from build123d import *

# Parameters (mm, degrees)
SKETCH1_W           = 15.875
SKETCH1_H           = 34.925
BOSS_EXTRUDE1_DEPTH = 6.35
SKETCH3_W           = 15.875
SKETCH3_H           = 18.415
BOSS_EXTRUDE2_DEPTH = 7.9375
SKETCH4_R           = 26.9875
CUT_EXTRUDE2_DEPTH  = 3.2385
SKETCH5_W           = 15.875
SKETCH5_H           = 8.68045
BOSS_EXTRUDE3_DEPTH = 3.175
FILLET1_R           = 0.254
FILLET2_R           = 3.175
SKETCH6_W           = 15.875
SKETCH6_H           = 6.35
BOSS_EXTRUDE4_DEPTH = 4.7625
SKETCH7_W           = 15.875
SKETCH7_H           = 3.175
BOSS_EXTRUDE5_DEPTH = 6.604
CUT_EXTRUDE3_REACH  = 48.174
SKETCH8_R           = 1.651


with BuildPart() as part:
    # Sketch1 → Boss-Extrude1 (new body)
    with BuildSketch(Plane.XY):
        with Locations((7.9375, 17.4625)):
            Rectangle(SKETCH1_W, SKETCH1_H)
    extrude(amount=BOSS_EXTRUDE1_DEPTH)

    # Sketch3 → Boss-Extrude2 (add)
    with BuildSketch(Plane.XY.offset(6.35)):
        with Locations((7.9375, 25.7175)):
            Rectangle(SKETCH3_W, SKETCH3_H)
    extrude(amount=BOSS_EXTRUDE2_DEPTH)

    # Sketch4 → Cut-Extrude2 (cut, symmetric)
    with BuildSketch(Plane(origin=(0, 28.42895, 0), x_dir=(-1, 0, 0), z_dir=(0, -1, 0))):
        with Locations((-7.9375, -36.4998)):
            Circle(SKETCH4_R)
    extrude(amount=CUT_EXTRUDE2_DEPTH, both=True, mode=Mode.SUBTRACT)

    # Sketch5 → Boss-Extrude3 (add)
    with BuildSketch(Plane.XY.offset(14.2875)):
        with Locations((7.9375, 20.850225)):
            Rectangle(SKETCH5_W, SKETCH5_H)
    extrude(amount=BOSS_EXTRUDE3_DEPTH)

    # Fillet1
    fillet1_edges = [part.edges().sort_by_distance(p)[0] for p in [
        (0, 33.296225, 14.2875),
        (15.875, 33.296225, 14.2875),
        (7.9375, 31.66745, 14.2875),
        (15.875, 28.42895, 10.705978065),
        (0, 28.42895, 10.705978065),
        (0, 25.19045, 14.084239033),
        (15.875, 25.19045, 14.084239033),
        (0, 31.66745, 12.496739033),
        (15.875, 31.66745, 12.496739033),
        (7.9375, 25.19045, 17.4625),
    ]]
    fillet(fillet1_edges, radius=FILLET1_R)

    # Fillet2
    fillet2_edges = [part.edges().sort_by_distance(p)[0] for p in [
        (7.9375, 16.51, 6.35),
    ]]
    fillet(fillet2_edges, radius=FILLET2_R)

    # Sketch6 → Boss-Extrude4 (add)
    with BuildSketch(Plane.XZ):
        with Locations((7.9375, 3.175)):
            Rectangle(SKETCH6_W, SKETCH6_H)
    extrude(amount=BOSS_EXTRUDE4_DEPTH)

    # Sketch7 → Boss-Extrude5 (add)
    with BuildSketch(Plane.XY.offset(6.35)):
        with Locations((7.9375, -3.175)):
            Rectangle(SKETCH7_W, SKETCH7_H)
    extrude(amount=BOSS_EXTRUDE5_DEPTH)

    # Sketch8 → Cut-Extrude3 (cut, up to next)
    with BuildSketch(Plane.XZ.offset(4.7625), mode=Mode.PRIVATE) as cut_extrude3_sk1:
        with Locations(Location((7.9375, 9.8552, 0), (0, 0, 270))):
            Circle(SKETCH8_R)
    cut_extrude3_tool1 = extrude(cut_extrude3_sk1.sketch, amount=-CUT_EXTRUDE3_REACH, mode=Mode.PRIVATE) & part.part
    add(cut_extrude3_tool1.solids().sort_by_distance((7.9375, -4.7625, 9.8552))[0], mode=Mode.SUBTRACT)


solid = part.part
Can you work these out from the model? Positions are in its coordinate system, mm. A direction names the side the tool comes from. Round coordinates to 2 decimals unless told otherwise and drop trailing zeros. Loops run counter-clockwise (first coordinate to the right, second up) from the corner with the lowest first, then second, coordinate; pieces in that order, holes last. Notation, with made-up numbers: (70, -11.75) - (118, -11.75) arc R15 ccw to (118, 14.25) - close; hole circle Ø11 at (-5.75, 42). An arc over 180 degrees is marked (long way). Write item = value, one per line. Start each with the question number.
(1) If I drill on probe 1 along Y at (x, z) = (2.5, 10.25) (1 decimal); probe 2 along Y at (x, z) = (12.75, 14) (3 decimals); probe 3 along Y at (x, z) = (10.5, 15.5), over which ranges is the centre line in solid material (lowest first)? Write a range as [from, to].
(2) If we section it at A-A (z = 13.5): Please give me the cut outline in (x, y) (3 decimals), and give its area (3 significant figures).
(3) For P1, Ø3.5, axis at x = 9.5, y = 33, coming from the +Z side; P2, Ø1.6, axis at x = 6, y = -3.5, coming from the +Z side; P3, Ø10, axis at y = 2.5, z = 10, coming from the +X side (3 decimals); P4, Ø1, axis at x = 4, y = -0.5, coming from the +Z side, each with a flat end and sliding along its axis, tell me the tip position at first contact or that it passes through.
(4) If we section it at D-D (z = 16): Please give me the cut outline in (x, y) (3 decimals).
(5) For faces 1 (the face through (8, 6, 6.35)), 2 (the face through (8, 33, 14.288)), 3 (the face through (8, -3, 12.954)), 4 (the face through (7.829, 28.384, 9.513)), which set-ups out of +Z, -Z, +X, -X, +Y, -Y let a thin tool reach every point of the face, with its end or its side?
(6) If we mould it in two halves opening along Z, with no side actions, what happens to faces 5 (the face through (8, 15, 0)), 6 (the face through (8, 16.51, 13)), 7 (the face through (6.933, -3.197, 11.165))? For each: released by +Z, released by -Z, zero draft, split by the parting line, or undercut.
(7) If we section it at C-C (y = 27): Please give me the cut outline in (x, z) (1 decimal), and give its area (3 significant figures).
Ans:
q1.probe_1 = [-4.8, -1.6], [16.5, 25.2], [31.7, 34.9]
q1.probe_2 = [16.51, 25.19], [31.667, 34.925]
q1.probe_3 = [16.51, 25.19]
q2.outline = (0, 16.51) - (15.875, 16.51) - (15.875, 24.936) arc R0.254 ccw to (15.621, 25.19) - (0.254, 25.19) arc R0.254 ccw to (0, 24.936) - close; (0, 31.921) arc R0.254 ccw to (0.254, 31.667) - (15.621, 31.667) arc R0.254 ccw to (15.875, 31.921) - (15.875, 34.925) - (0, 34.925) - close
q2.area = 189 mm²
q3.P1 = 14.29
q3.P2 = 12.95
q3.P3 = 15.875
q3.P4 = 6.35
q4.outline = (0, 16.51) - (15.875, 16.51) - (15.875, 24.936) arc R0.254 ccw to (15.621, 25.19) - (0.254, 25.19) arc R0.254 ccw to (0, 24.936) - close
q5.face_1 = +Z, +X, -X
q5.face_2 = +Z, +X, -X, +Y
q5.face_3 = +Z, +X, -X, -Y
q5.face_4 = +Z
q6.face_5 = released by -Z
q6.face_6 = zero draft
q6.face_7 = undercut
q7.outline = (0, 0) - (15.9, 0) - (15.9, 10.4) arc R0.3 ccw to (15.5, 10.6) arc R27 cw to (0.3, 10.6) arc R0.3 ccw to (0, 10.4) - close
q7.area = 157 mm²
